Check sheet for the drawn part. Datum: minimum x, y, z corner. Units: mm. Round coordinates to 2 decimals unless told otherwise and drop trailing zeros. Write each loop counter-clockwise with the first axis right and the second up, starting at its lowest first coordinate (ties: lowest second). Pieces come first, ordered by that corner, then holes. Notation, with made-up numbers: M 59,36.5 L 102,36.5 A13 ccw 102,55.5 Z; hole C -7,65 d8. An arc over 180 degrees is marked long. Use a Markdown table: item, result.
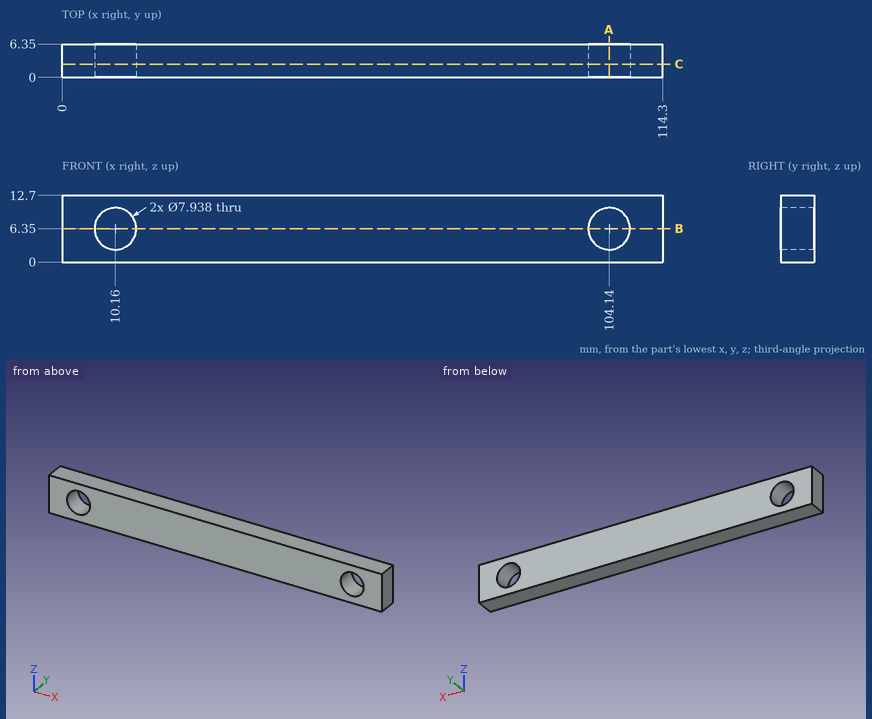
Item 1: Cross-section at A-A, the plane x = 104.14. Record the cut outline in (y, z).
Outcome:
| item | result |
|---|---|
| outline | M 0,0 L 6.35,0 L 6.35,2.38 L 0,2.38 Z; M 0,10.32 L 6.35,10.32 L 6.35,12.7 L 0,12.7 Z |
Item 2: Cross-section at C-C, the plane y = 2.5. Record the cut outline in (x, z), and give its area (3 significant figures).
Outcome:
| item | result |
|---|---|
| outline | M 0,0 L 114.3,0 L 114.3,12.7 L 0,12.7 Z; hole C 10.16,6.35 d7.94; hole C 104.14,6.35 d7.94 |
| area | 1,350 mm2 |
Item 3: Cross-section at B-B, the plane z = 6.35. Record the cut outline in (x, y).
Outcome:
| item | result |
|---|---|
| outline | M 0,0 L 6.19,0 L 6.19,6.35 L 0,6.35 Z; M 14.13,0 L 100.17,0 L 100.17,6.35 L 14.13,6.35 Z; M 108.11,0 L 114.3,0 L 114.3,6.35 L 108.11,6.35 Z |
Item 4: Go/stop test with a flat-tipped pin: pin 1 (1 mm diameter, centred on x = 90.5, y = 5.5, fed in from -Z). Record where the tip stops, or that it passes through.
Outcome:
| item | result |
|---|---|
| pin 1 | stops at z = 0 |
Item 5: Material ranges on line 1 along X through (y, z) = (1, 6.25); line 2 along Z through (x, y) = (10.16, 2.75); line 3 along X through (y, z) = (4.75, 3) (1 decimal), recorded low to high. Write a range as from..to.
Outcome:
| item | result |
|---|---|
| line 1 | x = 0..6.19, 14.13..100.17, 108.11..114.3 |
| line 2 | z = 0..2.38, 10.32..12.7 |
| line 3 | x = 0..8, 12.3..102, 106.3..114.3 |
